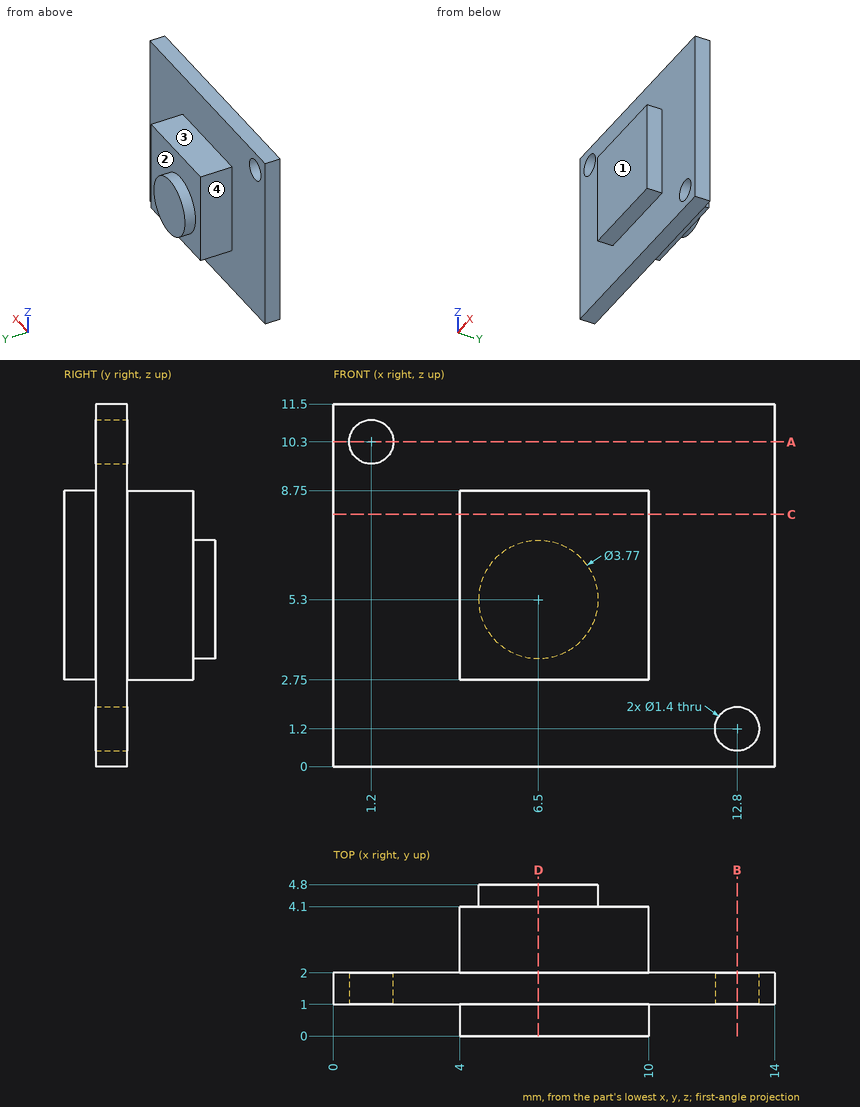
Here's the drawing with two shaded views (mm, measured from the low corner). I have some questions. A direction names the side the tool comes from. Round coordinates to 2 decimals unless told otherwise and drop trailing zeros. Write each loop counter-clockwise with the first axis right and the second up, starting at its lowest first coordinate (ties: lowest second). Pieces come first, ordered by that corner, then holes.
(1) Suppose I cut it at C-C on z = 8. Write out the boundary of the cut face in (x, y).
Findings below:
outline: (0, 1) - (4, 1) - (4, 0) - (10, 0) - (10, 1) - (14, 1) - (14, 2) - (10, 2) - (10, 4.1) - (4, 4.1) - (4, 2) - (0, 2) - close
(2) Which directions (+Z, -Z, +X, -X, +Y, -Y) give clear straight access to the entire face, cutting with the end or side of a thin tool? Please do the marked faces 1, 2, 3 and 4.
Findings below:
face 1: +Z, -Z, +X, -X, -Y
face 2: +Y
face 3: +Z, +X, -X, +Y
face 4: +Z, -Z, -X, +Y
(3) Suppose I cut it at D-D on x = 6.5. Write out the boundary of the cut face in (y, z) (3 decimals), and give its area (3 significant figures).
Findings below:
outline: (0, 2.75) - (1, 2.75) - (1, 0) - (2, 0) - (2, 2.75) - (4.1, 2.75) - (4.1, 3.415) - (4.8, 3.415) - (4.8, 7.185) - (4.1, 7.185) - (4.1, 8.75) - (2, 8.75) - (2, 11.5) - (1, 11.5) - (1, 8.75) - (0, 8.75) - close
area: 32.7 mm2
(4) For pin 1 (1.5 mm diameter, centred on x = 10, z = 5.5, fed in from +Y); pin 2 (0.5 mm diameter, centred on x = 8.5, y = 0.5, fed in from -Z); pin 3 (1.7 mm diameter, centred on y = 3.5, z = 5.5, fed in from +X); pin 4 (1.1 mm diameter, centred on x = 1.2, z = 10.3, fed in from -Y), each with a flat end and sliding along its axis, tell me the tip position at first contact or that it passes through.
Findings below:
pin 1: stops at y = 4.1
pin 2: stops at z = 2.75
pin 3: stops at x = 10
pin 4: passes through
(5) If I drill on probe 1 along Z at (x, y) = (12.8, 1.65); probe 2 along Y at (x, z) = (8.5, 7.5); probe 3 along Y at (x, z) = (5.25, 2.5), over which ranges is the centre line in solid material (lowest first)?
Findings below:
probe 1: z = 0 to 0.5, 1.9 to 11.5
probe 2: y = 0 to 4.1
probe 3: y = 1 to 2
(6) Suppose I cut it at B-B on x = 12.8. Write out the boundary of the cut face in (y, z), and give its area (3 significant figures).
Findings below:
outline: (1, 0) - (2, 0) - (2, 0.5) - (1, 0.5) - close; (1, 1.9) - (2, 1.9) - (2, 11.5) - (1, 11.5) - close
area: 10.1 mm2
(7) Suppose I cut it at A-A on z = 10.3. Write out the boundary of the cut face in (x, y).
Findings below:
outline: (0, 1) - (0.5, 1) - (0.5, 2) - (0, 2) - close; (1.9, 1) - (14, 1) - (14, 2) - (1.9, 2) - close
